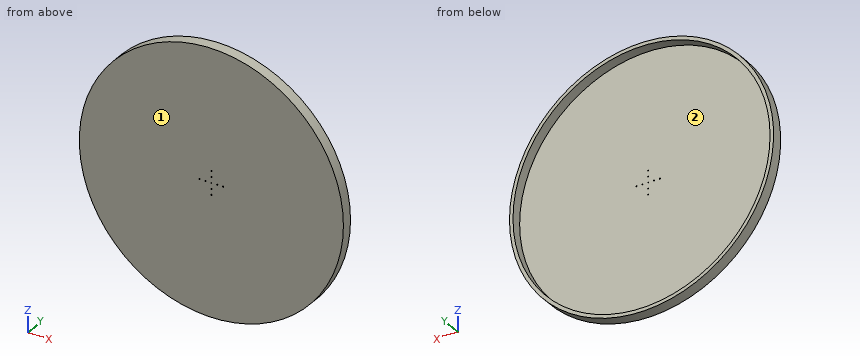
```python
from build123d import *

# Parameters (mm, degrees)
SKETCH1_R           = 472.5
BOSS_EXTRUDE1_DEPTH = 40
SKETCH3_R           = 460
CUT_EXTRUDE1_DEPTH  = 37.46
SKETCH5_R           = 1.5
CUT_EXTRUDE3_DEPTH  = 3.54
SKETCH8_R           = 2.02
CUT_EXTRUDE4_DEPTH  = 3.54


with BuildPart() as part:
    # Sketch1 → Boss-Extrude1 (new body)
    with BuildSketch(Plane(origin=(0, 0, 0), x_dir=(1, 0, 0), z_dir=(0, 1, 0))):
        Circle(SKETCH1_R)
    extrude(amount=BOSS_EXTRUDE1_DEPTH)

    # Sketch3 → Cut-Extrude1 (cut)
    with BuildSketch(Plane(origin=(0, 40, 0), x_dir=(1, 0, 0), z_dir=(0, 1, 0))):
        Circle(SKETCH3_R)
    extrude(amount=-CUT_EXTRUDE1_DEPTH, mode=Mode.SUBTRACT)

    # Sketch5 → Cut-Extrude3 (cut, through all)
    with BuildSketch(Plane(origin=(0, 2.54, 0), x_dir=(1, 0, 0), z_dir=(0, 1, 0))):
        Circle(SKETCH5_R)
    extrude(amount=-CUT_EXTRUDE3_DEPTH, mode=Mode.SUBTRACT)

    # Sketch8 → Cut-Extrude4 (cut, through all)
    with BuildSketch(Plane(origin=(0, 2.54, 0), x_dir=(1, 0, 0), z_dir=(0, 1, 0))):
        with Locations((0, 42)):
            Circle(SKETCH8_R)
        with Locations((42, 0)):
            Circle(SKETCH8_R)
        with Locations((0, -42)):
            Circle(SKETCH8_R)
        with Locations((-42, 0)):
            Circle(SKETCH8_R)
        with Locations((0, 21)):
            Circle(SKETCH8_R)
        with Locations((21, 0)):
            Circle(SKETCH8_R)
        with Locations((0, -21)):
            Circle(SKETCH8_R)
        with Locations((-21, 0)):
            Circle(SKETCH8_R)
    extrude(amount=-CUT_EXTRUDE4_DEPTH, mode=Mode.SUBTRACT)


solid = part.part
```
Verification items for the finished model (mm, model axes). Face numbers are marked on the shaded views. Coordinates: 2 decimals unless noted, no trailing zeros. Write each loop counter-clockwise with the first axis right and the second up, starting at its lowest first coordinate (ties: lowest second). Pieces come first, ordered by that corner, then holes. Notation, with made-up numbers: M 26.5,11.5 L 58.5,11.5 A31 ccw 58.5,42.5 Z; hole C 52.25,-4 d3. An arc over 180 degrees is marked long. Answer as a JSON object with one key per item and string values. Group by question number.
(1) Cross-section at C-C, the plane x = 232. Record the cut outline in (y, z), and give its area (3 significant figures).
(2) Material ranges on line 1 (X direction, y = 1, z = 0); line 2 (Z direction, x = 11, y = 34.5), recorded low to high.
(3) Gauge pin test, flat ends, axial feed: pin 1 (1.5 mm diameter, centred on x = -334, z = 94, fed in from +Y); pin 2 (3.5 mm diameter, centred on x = 0, z = -42, fed in from +Y); pin 3 (12 mm diameter, centred on y = 33, z = -220, fed in from +X); pin 4 (5 mm diameter, centred on x = -286.5, y = 25.5, fed in from -Z). Record the tip position at first contact, or that the pin passes through.
(4) Cross-section at B-B, the plane z = -206.5. Record the cut outline in (x, y), and give its area (3 significant figures).
(5) Cross-section at A-A, the plane y = 20. Record the cut outline in (x, z), and give its area (3 significant figures).
(6) Release check for a two-part mould opening along X. For the marked faces 1 and 2 record: +X half, -X half, draft (parallel to the pull), parting line (faces both ways), or undercut.
Reply:
{
 "1": {"outline": "M 0,-411.62 L 40,-411.62 L 40,-397.21 L 2.54,-397.21 L 2.54,397.21 L 40,397.21 L 40,411.62 L 0,411.62 Z", "area": "3,170 mm²"},
 "2": {"line 1": "-472.5 to -44.02, -39.98 to -23.02, -18.98 to -1.5, 1.5 to 18.98, 23.02 to 39.98, 44.02 to 472.5", "line 2": "-472.37 to -459.87, 459.87 to 472.37"},
 "3": {"pin 1": "y = 2.54", "pin 2": "through", "pin 3": "x = 421.26", "pin 4": "z = -377.62"},
 "4": {"outline": "M -424.99,0 L 424.99,0 L 424.99,40 L 411.04,40 L 411.04,2.54 L -411.04,2.54 L -411.04,40 L -424.99,40 Z", "area": "3,200 mm²"},
 "5": {"outline": "C 0,0 d945; hole C 0,0 d920", "area": "36,600 mm²"},
 "6": {"face 1": "draft", "face 2": "undercut"}
}
